Design review of the part built by this model. Coordinates are the model's own, in mm. Give positions to 0.01 mm unless a question says otherwise; leave off trailing zeros. Order: outer loops, then holes, each group sorted by start corner. A loop starts at its lowest first (then second) coordinate and runs counter-clockwise, first axis right, second up. Notation, with made-up numbers: (14, 9) -> (32, 9) arc R9 cw to (32, 25) -> close; hole circle Ø2 at (47.5, 24.25). An arc over 180 degrees is marked (long way). Return JSON: item names as keys, results as strings.
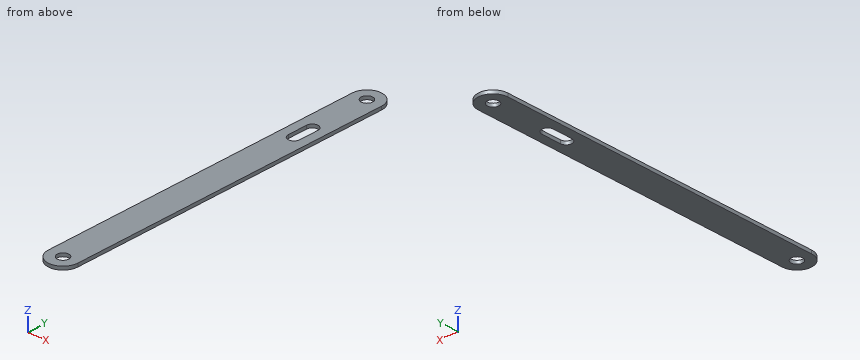
Autodesk Inventor part; units mm, degrees
ref_plane "YZ Plane" through (0, 0, 0) normal (1, 0, 0) x (0, 1, 0)
ref_plane "XZ Plane" through (0, 0, 0) normal (0, 1, 0) x (-1, 0, 0)
ref_plane "XY Plane" through (0, 0, 0) normal (0, 0, 1) x (1, 0, 0)
sketch "スケッチ1" plane through (0, 0, 0) normal (0, 0, 1) x (1, 0, 0)
  line L0 (18, 0) -> (18, 200)
  line L1 (0, 200) -> (0, 0)
  line L2 (9, 200) -> (9, 0) construction
  arc A0 (18, 200) -> (0, 200) centre (9, 200) ccw
  arc A1 (0, 0) -> (18, 0) centre (9, 0) ccw
  circle A2 centre (9, 0) radius 3.5
  circle A3 centre (9, 200) radius 3.5
  dimension "d35" = 18
  dimension "d36" = 200
  dimension "d37" = 7
  dimension "d38" = 7
extrude "押し出し1" add sketch "スケッチ1" along normal blind 2
sketch "スケッチ3" plane through (0, 0, 2) normal (0, 0, 1) x (1, 0, 0)
  circle A0 centre (9, 0) radius 3.5
  circle A1 centre (9, 200) radius 3.5
  arc A2 (18, 200) -> (0, 200) centre (9, 200) ccw
  line L0 (0, 200) -> (0, 0)
  arc A3 (0, 0) -> (18, 0) centre (9, 0) ccw
  line L1 (18, 0) -> (18, 200)
  circle A4 centre (9, 0) radius 3.5
  line L2 (9, 200) -> (9, 0) construction
  arc A5 (5.5, 152) -> (12.5, 152) centre (9, 152) ccw
  arc A6 (12.5, 164) -> (5.5, 164) centre (9, 164) ccw
  line L3 (5.5, 164) -> (5.5, 152)
  line L4 (12.5, 164) -> (12.5, 152)
  dimension "d41" = 7
  dimension "d42" = 48
  dimension "d43" = 7
  dimension "d44" = 36
extrude "押し出し2" cut sketch "スケッチ3" against normal through all contours L3 A6 L4 A5
properties part number "foot_link_lever" material "GFRP"
Item 1: Add section B-B (z = 1.4). Give the boundary of the cut face in (x, y).
Result set:
{"outline": "(0, 0) arc R9 ccw to (18, 0) -> (18, 200) arc R9 ccw to (0, 200) -> close; hole circle Ø7 at (9, 0); hole (5.5, 152) arc R3.5 ccw to (12.5, 152) -> (12.5, 164) arc R3.5 ccw to (5.5, 164) -> close; hole circle Ø7 at (9, 200)"}
Item 2: Add section A-A (x = 9.25). Give the boundary of the cut face in (y, z).
Result set:
{"outline": "(-9, 0) -> (-3.49, 0) -> (-3.49, 2) -> (-9, 2) -> close; (3.49, 0) -> (148.51, 0) -> (148.51, 2) -> (3.49, 2) -> close; (167.49, 0) -> (196.51, 0) -> (196.51, 2) -> (167.49, 2) -> close; (203.49, 0) -> (209, 0) -> (209, 2) -> (203.49, 2) -> close"}
Item 3: Wall thickness on L1, parallel to Y at x = 9, z = 1.55; L2, parallel to Y at x = 8.25, z = 0.35; L3, parallel to X at y = 200, z = 0.95: over which ranges is each line inside the solid? List them lowest first. Write a range as [from, to].
Result set:
{"L1": "y = [-9, -3.5], [3.5, 148.5], [167.5, 196.5], [203.5, 209]", "L2": "y = [-8.97, -3.42], [3.42, 148.58], [167.42, 196.58], [203.42, 208.97]", "L3": "x = [0, 5.5], [12.5, 18]"}
Item 4: For pin 1 (6.5 mm diameter, centred on x = 9, y = 0, fed in from +Z), flat-tipped, find the tip position at first contact; note if it passes through.
Result set:
{"pin 1": "passes through"}
